from build123d import *

# Parameters (mm, degrees)
SKETCH1_R           = 45
BOSS_EXTRUDE1_DEPTH = 275
FILLET1_R           = 10
CHAMFER1_SIZE       = 150
CHAMFER1_SIZE2      = 26.449047106
FILLET2_R           = 100
CHAMFER2_SIZE       = 40
CHAMFER2_SIZE2      = 6.617933019
FILLET3_R           = 70
SKETCH2_R           = 15
BOSS_EXTRUDE2_DEPTH = 25


with BuildPart() as part:
    # Sketch1 → Boss-Extrude1 (new body)
    with BuildSketch(Plane(origin=(0, 0, 0), x_dir=(1, 0, 0), z_dir=(0, 1, 0))):
        with Locations(Location((0, 0, 0), (0, 0, 270))):
            Circle(SKETCH1_R)
    extrude(amount=BOSS_EXTRUDE1_DEPTH)

    # Fillet1
    fillet1_edges = [part.edges().sort_by_distance(p)[0] for p in [
        (0, 0, -45),
    ]]
    fillet(fillet1_edges, radius=FILLET1_R)

    # Chamfer1
    chamfer1_edges = [part.edges().sort_by_distance(p)[0] for p in [
        (0, 275, -45),
    ]]
    chamfer1_side = [part.faces().sort_by_distance(p)[0] for p in [
        (0, 142.5, -45),
    ]]
    chamfer(chamfer1_edges, length=CHAMFER1_SIZE, length2=CHAMFER1_SIZE2, reference=chamfer1_side[0])

    # Fillet2
    fillet2_edges = [part.edges().sort_by_distance(p)[0] for p in [
        (0, 125, -45),
    ]]
    fillet(fillet2_edges, radius=FILLET2_R)

    # Chamfer2
    chamfer2_edges = [part.edges().sort_by_distance(p)[0] for p in [
        (0, 275, -18.550952894),
    ]]
    chamfer2_side = [part.faces().sort_by_distance(p)[0] for p in [
        (0, 204.307975707, -31.015864097),
    ]]
    chamfer(chamfer2_edges, length=CHAMFER2_SIZE, length2=CHAMFER2_SIZE2, reference=chamfer2_side[0])

    # Fillet3
    fillet3_edges = [part.edges().sort_by_distance(p)[0] for p in [
        (0, 235.60768988, -25.49688),
    ]]
    fillet(fillet3_edges, radius=FILLET3_R)

    # Sketch2 → Boss-Extrude2 (add)
    with BuildSketch(Plane(origin=(0, 275, 0), x_dir=(1, 0, 0), z_dir=(0, 1, 0))):
        with Locations(Location((0, 0, 0), (0, 0, 270))):
            Circle(SKETCH2_R)
    extrude(amount=BOSS_EXTRUDE2_DEPTH)


solid = part.part
Design review of the part built by this model. Coordinates are the model's own, in mm. A direction names the side the tool comes from. Give positions to 0.01 mm unless a question says otherwise; leave off trailing zeros. Loops run counter-clockwise (first coordinate to the right, second up) from the corner with the lowest first, then second, coordinate; pieces in that order, holes last. Notation, with made-up numbers: (60, -39) - (68, -39) arc R30 ccw to (68, -11) - close; hole circle Ø10 at (66, 76.25). An arc over 180 degrees is marked (long way). Write item = value, one per line.
1) Clearance check with flat-ended pins moving along their axes: pin 1 Ø3 at (x, y) = (31, 162) entering from -Z; pin 2 Ø1.5 at (y, z) = (92, -14.5) entering from -X; pin 3 Ø5 at (y, z) = (73, -22.5) entering from -X. State where each tip first meets the part, or that it passes through.
Result sheet:
pin_1 = -24.75
pin_2 = -42.85
pin_3 = -40.31
2) To check wall thickness, follow line 1 (X direction, y = 105.5, z = -17); line 2 (Z direction, x = -15.5, y = 70); line 3 (Z direction, x = 6, y = 105). State the ranges of each line that lie inside material, in increasing order.
Result sheet:
line_1 = -41.67 to 41.67
line_2 = -42.25 to 42.25
line_3 = -44.6 to 44.6
3) Take a section at B-B on y = 64.5. State the section outline as (x, z) points, and give its area (3 significant figures).
Result sheet:
outline = circle Ø90 at (0, 0)
area = 6,360 mm2
4) Tool access review of faces 1 (the face through (0.66, 287.325, -14.985)), 2 (the face through (0, 300, 0)), 3 (the face through (-7, 275, -10)): name each direction out of +Z, -Z, +X, -X, +Y, -Y from which nothing blocks a thin tool from reaching the whole face with its end or side.
Result sheet:
face_1 = +Y
face_2 = +Z, -Z, +X, -X, +Y
face_3 = none
5) Take a section at A-A on y = 136.5. State the section outline as (x, z) points, and give its area (3 significant figures).
Result sheet:
outline = circle Ø85.94 at (0, 0)
area = 5,800 mm2
